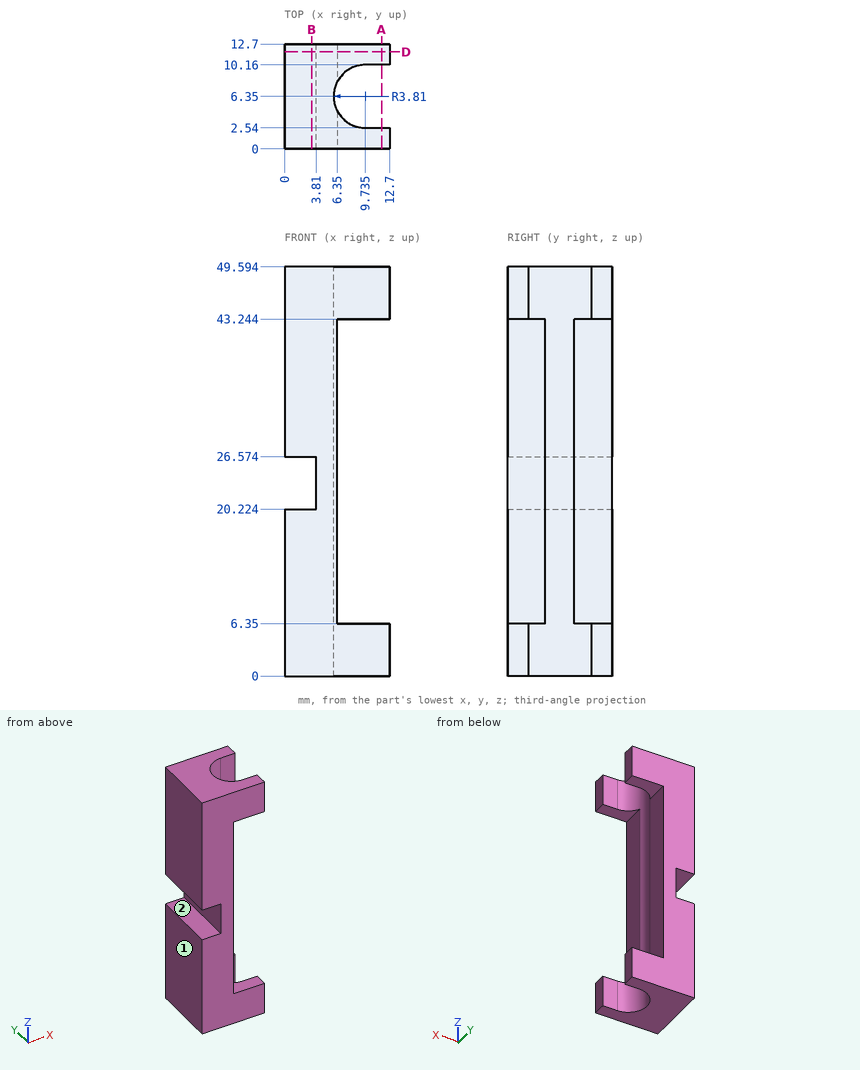
Source: three-view drawing plus pictorial views. Frame: mm from the lowest corner of the part. A direction names the side the tool comes from. Round coordinates to 2 decimals unless told otherwise and drop trailing zeros. Write each loop counter-clockwise with the first axis right and the second up, starting at its lowest first coordinate (ties: lowest second). Pieces come first, ordered by that corner, then holes. Notation, with made-up numbers: M -2.75,-35.75 L 25.25,-35.75 A14 cw 25.25,-22.75 Z; hole C 62.5,-39 d2. An arc over 180 degrees is marked long. One line per item, written item: value. Start each with the question number.
Item 1: Set-up query: the marked faces 1 and 2. Return all of +Z, -Z, +X, -X, +Y, -Y with unobstructed straight access to the full face (end or side cutting, diameter ignored); none if empty.
Item 2: Pin query (flat end, axial travel): pin 1 (2 mm diameter, centred on x = 7.5, z = 22.5, fed in from -Y); pin 2 (5 mm diameter, centred on x = 11, y = 9.5, fed in from +Z); pin 3 (1.4 mm diameter, centred on y = 11, z = 29.5, fed in from +X). Return the tip coordinate at first contact, or that it passes through.
Item 3: Ray query, L1, parallel to Z at x = 1.5, y = 11.25; L2, parallel to Z at x = 8.5, y = 12.25; L3, parallel to Y at x = 10.25, z = 4. Return the intervals inside material, ascending. Write a range as from..to.
Item 4: Section query D-D (y = 11.75). Return the cut outline in (x, z), plus the area to 3 significant figures.
Item 5: Section query A-A (x = 11.75). Return the cut outline in (y, z).
Item 6: Section query B-B (x = 3.25). Return the cut outline in (y, z).
Result set:
1. face 1: +Z, -Z, -X, +Y, -Y
1. face 2: -X, +Y, -Y
2. pin 1: passes through
2. pin 2: stops at z = 49.59
2. pin 3: stops at x = 6.35
3. L1: z = 0..20.22, 26.57..49.59
3. L2: z = 0..6.35, 43.24..49.59
3. L3: y = 0..2.54, 10.16..12.7
4. outline: M 0,0 L 12.7,0 L 12.7,6.35 L 6.35,6.35 L 6.35,43.24 L 12.7,43.24 L 12.7,49.59 L 0,49.59 L 0,26.57 L 3.81,26.57 L 3.81,20.22 L 0,20.22 Z
4. area: 371 mm²
5. outline: M 0,0 L 2.54,0 L 2.54,6.35 L 0,6.35 Z; M 0,43.24 L 2.54,43.24 L 2.54,49.59 L 0,49.59 Z; M 10.16,0 L 12.7,0 L 12.7,6.35 L 10.16,6.35 Z; M 10.16,43.24 L 12.7,43.24 L 12.7,49.59 L 10.16,49.59 Z
6. outline: M 0,0 L 12.7,0 L 12.7,20.22 L 0,20.22 Z; M 0,26.57 L 12.7,26.57 L 12.7,49.59 L 0,49.59 Z
